Could you check a few things on this drawing? It's one solid part, dimensions in mm from its lowest x, y, z. Coordinates: 2 decimals unless noted, no trailing zeros. Order: outer loops, then holes, each group sorted by start corner. A loop starts at its lowest first (then second) coordinate and runs counter-clockwise, first axis right, second up. Notation, with made-up numbers: (6, 72) -> (14, 72) arc R21 cw to (14, 110) -> close; hole circle Ø11 at (60.25, -6.5). An arc over 180 degrees is marked (long way). Use a Markdown table: item, result. Add a question column.
1. Suppose I cut it at B-B, the plane x = 75. List the corners of the cut face in (y, z) for me, then the cut area to 4 significant figures.
2. Suppose I cut it at A-A, the plane y = 20. List the corners of the cut face in (x, z) for me.
3. If I drill on line 1 along Y through (x, z) = (75, 7); line 2 along Y through (x, z) = (25, 8); line 3 along X through (y, z) = (17, 2.25), over which ranges is the centre line in solid material (lowest first)? Write a range as from..to.
4. Suppose I cut it at C-C, the plane z = 6. List the corners of the cut face in (x, y) for me, then the cut area to 3 significant figures.
5. For pin 1 Ø2.5 at (x, y) = (53, 276.5) entering from +Z; pin 2 Ø6 at (x, y) = (44.5, 107.5) entering from -Z; pin 3 Ø2.5 at (y, z) = (277, 6) entering from -X; pin 4 Ø4 at (y, z) = (278, 5) entering from +X, each with a flat end and sliding along its axis, tell me the tip position at first contact or that it passes through.
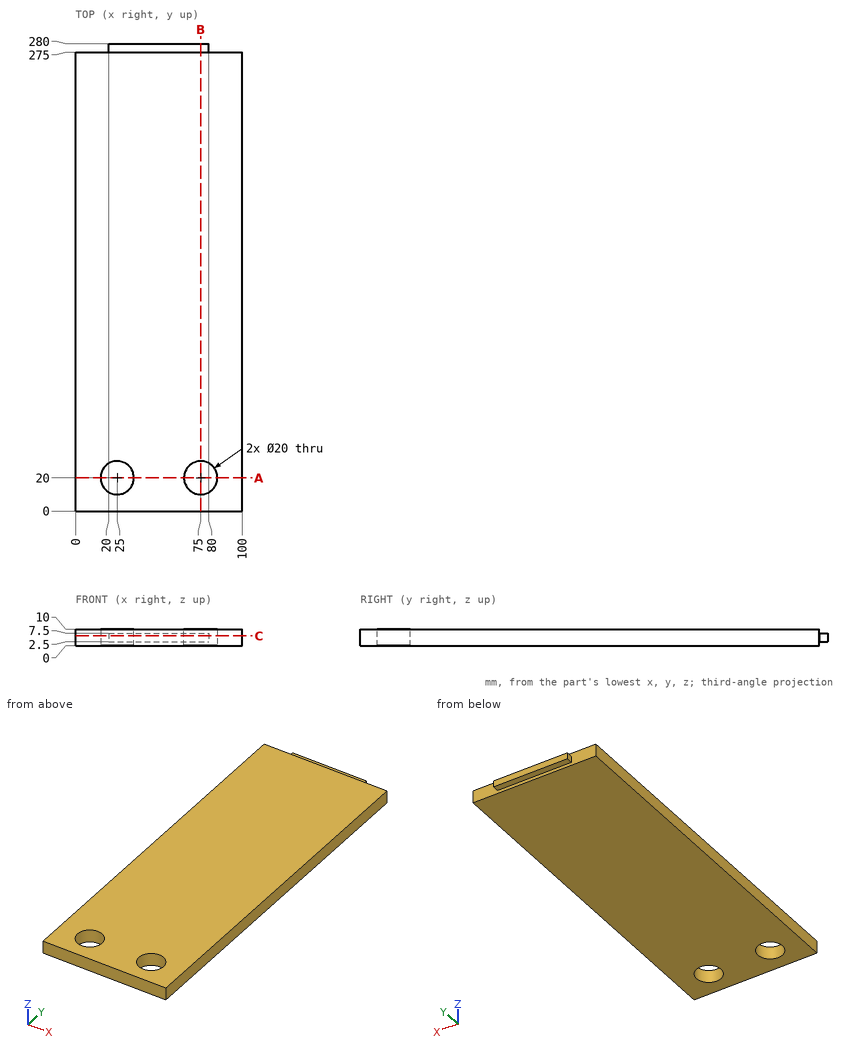
Worked out:
| question | item | result |
|---|---|---|
| 1 | outline | (0, 0) -> (10, 0) -> (10, 10) -> (0, 10) -> close; (30, 0) -> (275, 0) -> (275, 2.5) -> (280, 2.5) -> (280, 7.5) -> (275, 7.5) -> (275, 10) -> (30, 10) -> close |
| 1 | area | 2,575 mm² |
| 2 | outline | (0, 0) -> (15, 0) -> (15, 10) -> (0, 10) -> close; (35, 0) -> (65, 0) -> (65, 10) -> (35, 10) -> close; (85, 0) -> (100, 0) -> (100, 10) -> (85, 10) -> close |
| 3 | line 1 | y = 0..10, 30..280 |
| 3 | line 2 | y = 0..10, 30..275 |
| 3 | line 3 | x = 0..15.46, 34.54..65.46, 84.54..100 |
| 4 | outline | (0, 0) -> (100, 0) -> (100, 275) -> (80, 275) -> (80, 280) -> (20, 280) -> (20, 275) -> (0, 275) -> close; hole circle Ø20 at (25, 20); hole circle Ø20 at (75, 20) |
| 4 | area | 27,200 mm² |
| 5 | pin 1 | stops at z = 7.5 |
| 5 | pin 2 | stops at z = 0 |
| 5 | pin 3 | stops at x = 20 |
| 5 | pin 4 | stops at x = 80 |
